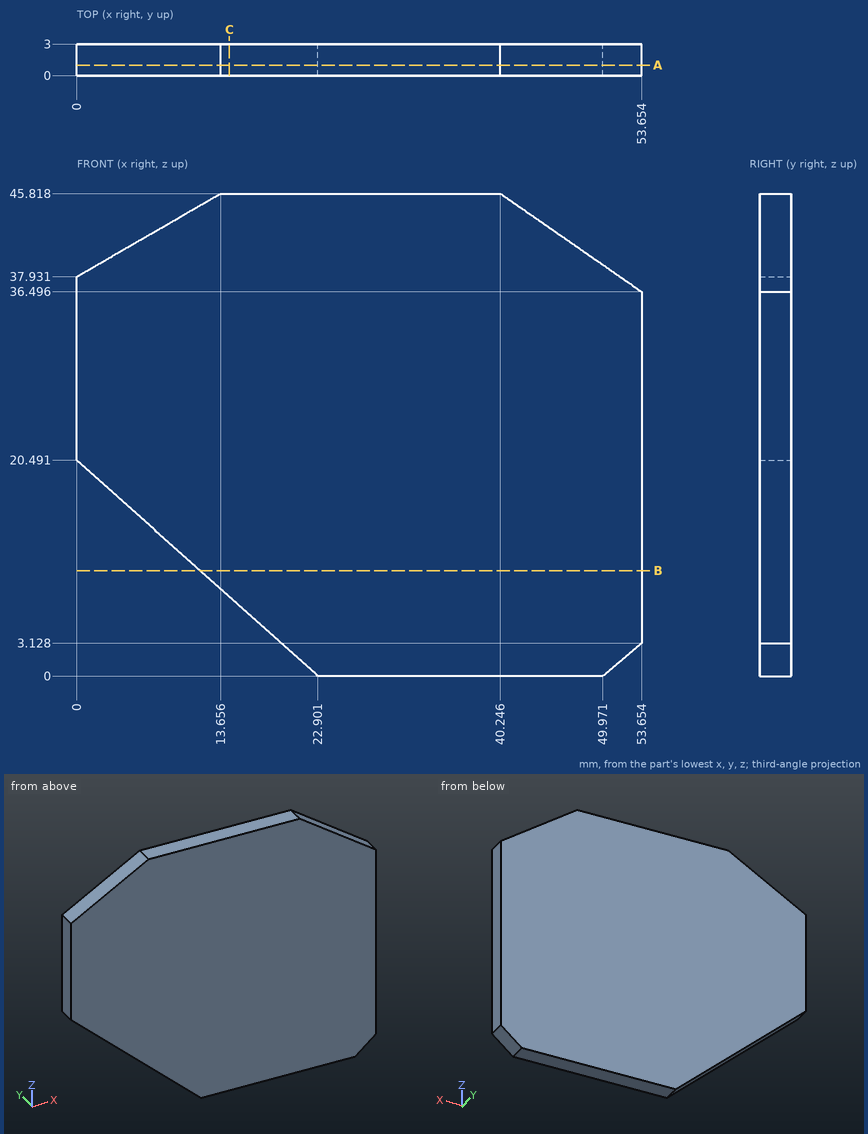
Design review of the part shown in the three views and the two pictorial views. Dimensions are in mm from the part's minimum x, y and z. Round coordinates to 2 decimals unless told otherwise and drop trailing zeros. Loops run counter-clockwise (first coordinate to the right, second up) from the corner with the lowest first, then second, coordinate; pieces in that order, holes last. Notation, with made-up numbers: (-28.5, 42) -> (-9.5, 42) arc R13 cw to (-9.5, 60) -> close; hole circle Ø6 at (45, 43.25). An arc over 180 degrees is marked (long way). Return JSON: item names as keys, results as strings.
(1) Add section A-A on y = 1. Write out the cut boundary in (x, z) (1 decimal), plus the area to 3 significant figures.
Solved:
{"outline": "(0, 20.5) -> (22.9, 0) -> (50, 0) -> (53.7, 3.1) -> (53.7, 36.5) -> (40.2, 45.8) -> (13.7, 45.8) -> (0, 37.9) -> close", "area": "2,100 mm2"}
(2) For line 1 (Z direction, x = 9, y = 1.7); line 2 (X direction, y = 2.3, z = 8) (1 decimal); line 3 (Z direction, x = 42, y = 1.85), list the stretches that pass through material, from the lowest coordinate up.
Solved:
{"line 1": "12.44 to 43.13", "line 2": "14 to 53.7", "line 3": "0 to 44.6"}
(3) Add section C-C on x = 14.5. Write out the cut boundary in (y, z).
Solved:
{"outline": "(0, 7.52) -> (3, 7.52) -> (3, 45.82) -> (0, 45.82) -> close"}
(4) Add section B-B on z = 10. Write out the cut boundary in (x, y) (1 decimal), plus the area to 3 significant figures.
Solved:
{"outline": "(11.7, 0) -> (53.7, 0) -> (53.7, 3) -> (11.7, 3) -> close", "area": "126 mm2"}
